Could you check a few things on this drawing? It's one solid part, dimensions in mm from its lowest x, y, z. Give positions to 0.01 mm unless a question says otherwise; leave off trailing zeros. Loops run counter-clockwise (first coordinate to the right, second up) from the corner with the lowest first, then second, coordinate; pieces in that order, holes last. Notation, with made-up numbers: M 19,-6.75 L 34,-6.75 A21 cw 34,24.25 Z; hole C 86,50.5 d7. An arc over 180 degrees is marked long. Answer as a JSON object with one key per item and string values.
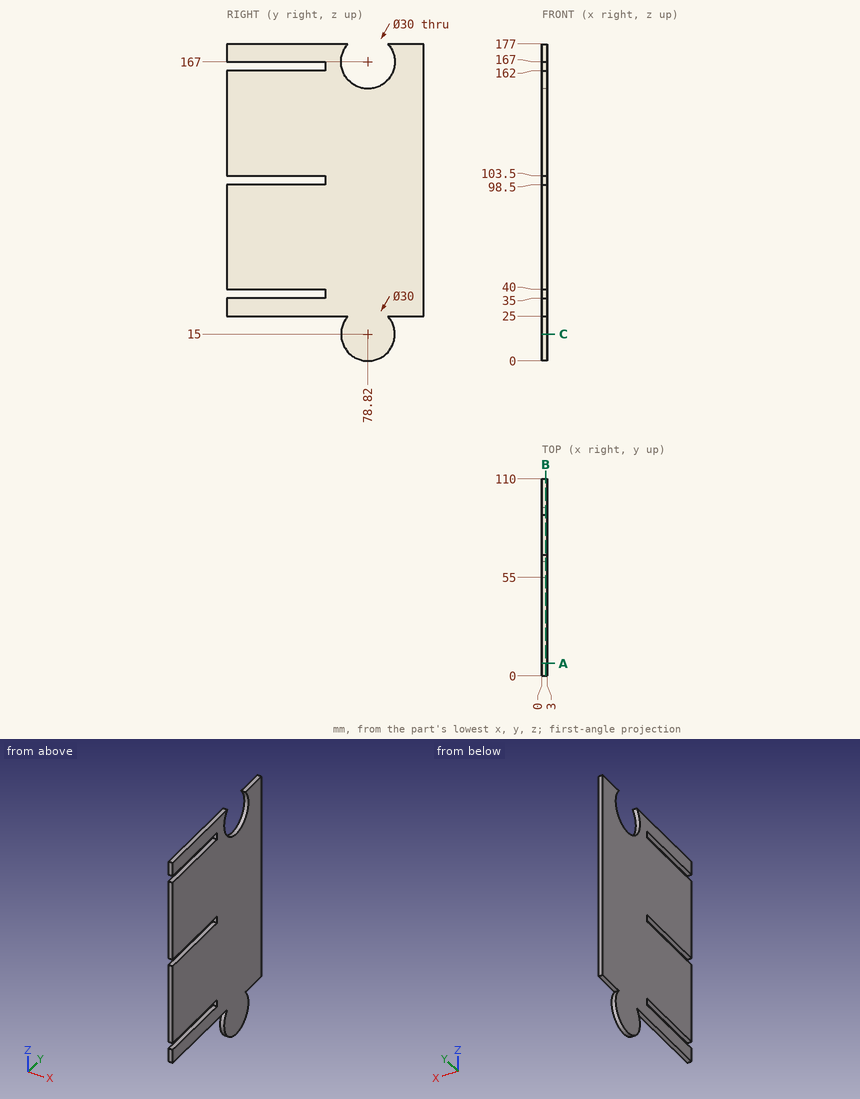
1) Suppose I cut it at A-A, the plane y = 7. Write out the boundary of the cut face in (x, z), and give its area (3 significant figures).
Answer list:
{"outline": "M 0,25 L 3,25 L 3,35 L 0,35 Z; M 0,40 L 3,40 L 3,98.5 L 0,98.5 Z; M 0,103.5 L 3,103.5 L 3,162 L 0,162 Z; M 0,167 L 3,167 L 3,177 L 0,177 Z", "area": "411 mm^2"}
2) Please list where these lines run through material, in increasing order: line 1 along Z through (x, y) = (1.6, 50.5); line 2 along Z through (x, y) = (1.15, 78.5); line 3 along Z through (x, y) = (2.85, 67.5). Write a range as from..to.
Answer list:
{"line 1": "25..35, 40..98.5, 103.5..162, 167..177", "line 2": "0..152", "line 3": "5.16..24.84, 25..157.16, 176.84..177"}
3) Will these pins go through, and if not, where does the flat tip stop? pin 1 Ø0.9 at (x, z) = (1, 165.5) entering from -Y; pin 2 Ø1.5 at (x, y) = (2, 27) entering from -Z; pin 3 Ø24 at (y, z) = (78.82, 167) entering from +X.
Answer list:
{"pin 1": "y = 55", "pin 2": "z = 25", "pin 3": "through"}
4) Suppose I cut it at B-B, the plane x = 2.1. Write out the boundary of the cut face in (y, z).
Answer list:
{"outline": "M 0,25 L 67.64,25 A15 ccw long 90,25 L 110,25 L 110,177 L 90,177 A15 cw long 67.64,177 L 0,177 L 0,167 L 55,167 L 55,162 L 0,162 L 0,103.5 L 55,103.5 L 55,98.5 L 0,98.5 L 0,40 L 55,40 L 55,35 L 0,35 Z"}
5) Suppose I cut it at C-C, the plane z = 15. Write out the boundary of the cut face in (x, y).
Answer list:
{"outline": "M 0,63.82 L 3,63.82 L 3,93.82 L 0,93.82 Z"}
